```python
from build123d import *

# Parameters (mm, degrees)
SKETCH1_W           = 203.2
SKETCH1_H           = 247.65
BOSS_EXTRUDE1_DEPTH = 19.05
FILLET1_R           = 7.62
SHELL1_T            = -2.54
CUT_EXTRUDE1_REACH  = 163.301
SKETCH2_W           = 130.745
SKETCH2_H           = 180.34
FILLET2_R           = 2.54
CUT_EXTRUDE2_REACH  = 163.301
SKETCH3_R           = 2.54
SKETCH4_W           = 135.825
SKETCH4_H           = 185.42
CUT_EXTRUDE3_DEPTH  = 1.27


with BuildPart() as part:
    # Sketch1 → Boss-Extrude1 (new body)
    with BuildSketch(Plane(origin=(0, 0, 0), x_dir=(1, 0, 0), z_dir=(0, 1, 0))):
        Rectangle(SKETCH1_W, SKETCH1_H)
    extrude(amount=BOSS_EXTRUDE1_DEPTH)

    # Fillet1
    fillet1_edges = [part.edges().sort_by_distance(p)[0] for p in [
        (-101.6, 19.05, 0),
        (0, 19.05, 123.825),
        (101.6, 19.05, 0),
        (0, 19.05, -123.825),
    ]]
    fillet(fillet1_edges, radius=FILLET1_R)

    # Shell1
    shell1_openings = [part.faces().sort_by_distance(p)[0] for p in [
        (0, 0, 0),
    ]]
    offset(amount=SHELL1_T, openings=shell1_openings)

    # Sketch2 → Cut-Extrude1 (cut, up to next)
    with BuildSketch(Plane(origin=(0, 19.05, 0), x_dir=(1, 0, 0), z_dir=(0, 1, 0)), mode=Mode.PRIVATE) as cut_extrude1_sk1:
        with Locations((2.5725, 0)):
            Rectangle(SKETCH2_W, SKETCH2_H)
    cut_extrude1_tool1 = extrude(cut_extrude1_sk1.sketch, amount=-CUT_EXTRUDE1_REACH, mode=Mode.PRIVATE) & part.part
    add(cut_extrude1_tool1.solids().sort_by_distance((2.5725, 19.05, 0))[0], mode=Mode.SUBTRACT)

    # Fillet2
    fillet2_edges = [part.edges().sort_by_distance(p)[0] for p in [
        (-62.8, 19.05, 0),
        (2.5725, 19.05, 90.17),
        (67.945, 19.05, 0),
        (2.5725, 19.05, -90.17),
    ]]
    fillet(fillet2_edges, radius=FILLET2_R - 0.0001)  # a hair under: the kernel refuses the full size

    # Sketch3 → Cut-Extrude2 (cut, up to next)
    with BuildSketch(Plane(origin=(0, 19.05, 0), x_dir=(1, 0, 0), z_dir=(0, 1, 0)), mode=Mode.PRIVATE) as cut_extrude2_sk1:
        with Locations(Location((-85.725, 104.775, 0), (0, 0, 270))):
            Circle(SKETCH3_R)
    cut_extrude2_tool1 = extrude(cut_extrude2_sk1.sketch, amount=-CUT_EXTRUDE2_REACH, mode=Mode.PRIVATE) & part.part
    # Sketch3 → Cut-Extrude2 (cut, up to next)
    with BuildSketch(Plane(origin=(0, 19.05, 0), x_dir=(1, 0, 0), z_dir=(0, 1, 0)), mode=Mode.PRIVATE) as cut_extrude2_sk2:
        with Locations(Location((-85.725, -104.775, 0), (0, 0, 270))):
            Circle(SKETCH3_R)
    cut_extrude2_tool2 = extrude(cut_extrude2_sk2.sketch, amount=-CUT_EXTRUDE2_REACH, mode=Mode.PRIVATE) & part.part
    add(cut_extrude2_tool1.solids().sort_by_distance((-85.725, 19.05, -104.775))[0], mode=Mode.SUBTRACT)
    add(cut_extrude2_tool2.solids().sort_by_distance((-85.725, 19.05, 104.775))[0], mode=Mode.SUBTRACT)

    # Sketch4 → Cut-Extrude3 (cut)
    with BuildSketch(Plane.XZ.offset(-16.51)):
        with Locations((2.5725, 0)):
            Rectangle(SKETCH4_W, SKETCH4_H)
    extrude(amount=-CUT_EXTRUDE3_DEPTH, mode=Mode.SUBTRACT)


solid = part.part
```
Input: part model. Units: mm. Frame: model coordinates. A direction names the side the tool comes from. Coordinates: 2 decimals unless noted, no trailing zeros. Write each loop counter-clockwise with the first axis right and the second up, starting at its lowest first coordinate (ties: lowest second). Pieces come first, ordered by that corner, then holes. Notation, with made-up numbers: (27.5, -22) -> (47.5, -22) arc R27 cw to (47.5, 11) -> close; hole circle Ø5 at (47, -18). An arc over 180 degrees is marked (long way). Write each question's results on one line, items separated by ' | '.
Item 1: Section query B-B on y = 3. Return loops of the section in (x, z) (3 decimals).
Conclusion:
outline: (-101.6, -123.825) -> (101.6, -123.825) -> (101.6, 123.825) -> (-101.6, 123.825) -> close; hole (-99.06, -121.285) -> (99.06, -121.285) -> (99.06, 121.285) -> (-99.06, 121.285) -> close
Item 2: Section query C-C on x = -5. Return loops of the section in (y, z) (3 decimals), plus the area to 3 significant figures.
Conclusion:
outline: (0, -123.825) -> (11.43, -123.825) arc R7.62 ccw to (19.05, -116.205) -> (19.05, -92.71) arc R2.54 ccw to (17.78, -90.51) -> (17.78, -92.71) -> (16.51, -92.71) -> (16.51, -116.205) arc R5.08 cw to (11.43, -121.285) -> (0, -121.285) -> close; (0, 121.285) -> (11.43, 121.285) arc R5.08 cw to (16.51, 116.205) -> (16.51, 92.71) -> (17.78, 92.71) -> (17.78, 90.51) arc R2.54 ccw to (19.05, 92.71) -> (19.05, 116.205) arc R7.62 ccw to (11.43, 123.825) -> (0, 123.825) -> close | area: 232 mm^2
Item 3: Material intervals for probe 1 along X at (y, z) = (6, 113); probe 2 along Z at (x, y) = (86, 11) (3 decimals); probe 3 along Y at (x, z) = (27.5, 98), sorted ascending.
Conclusion:
probe 1: x = -101.6 to -99.06, 99.06 to 101.6 | probe 2: z = -123.825 to -121.285, 121.285 to 123.825 | probe 3: y = 16.51 to 19.05
Item 4: Mould query, pull axis X, two halves, no side actions, for faces 1 (the flat face through (-99.06, 6, 2)), 2 (the flat face through (-1, 6, -121.285)), 3 (the flat face through (-101.6, 6, 2)), 4 (the cylindrical face through (1.42, 16.76, -121.65)). Classes: +X half, -X half, draft (parallel to the pull), parting line (faces both ways), or undercut.
Conclusion:
face 1: undercut | face 2: undercut | face 3: -X half | face 4: draft
Item 5: Pin query (flat end, axial travel): pin 1 Ø3 at (x, z) = (-85.725, -104.775) entering from +Y; pin 2 Ø0.6 at (x, y) = (-2, 17) entering from +Z; pin 3 Ø1.4 at (y, z) = (17.5, -3) entering from -X; pin 4 Ø3 at (x, y) = (4.5, 14) entering from +Z. Return the tip coordinate at first contact, or that it passes through.
Conclusion:
pin 1: passes through | pin 2: stops at z = 121.71 | pin 3: stops at x = -99.39 | pin 4: stops at z = 123.75
Item 6: Section query A-A on z = -15.5. Return loops of the section in (x, y) (3 decimals).
Conclusion:
outline: (-101.6, 0) -> (-99.06, 0) -> (-99.06, 11.43) arc R5.08 cw to (-93.98, 16.51) -> (-65.34, 16.51) -> (-65.34, 17.78) -> (-63.14, 17.78) arc R2.54 ccw to (-65.34, 19.05) -> (-93.98, 19.05) arc R7.62 ccw to (-101.6, 11.43) -> close; (68.285, 17.78) -> (70.485, 17.78) -> (70.485, 16.51) -> (93.98, 16.51) arc R5.08 cw to (99.06, 11.43) -> (99.06, 0) -> (101.6, 0) -> (101.6, 11.43) arc R7.62 ccw to (93.98, 19.05) -> (70.485, 19.05) arc R2.54 ccw to start
Item 7: Set-up query: faces 5 (the flat face through (99.06, 6, 2)), 6 (the cylindrical face through (-99.427, 16.759, -1.734)). Return all of +Z, -Z, +X, -X, +Y, -Y with unobstructed straight access to the full face (end or side cutting, diameter ignored); none if empty.
Conclusion:
face 5: -Y | face 6: +Z, -Z, -X, +Y
Item 8: Section query D-D on x = 77. Return loops of the section in (y, z) (3 decimals).
Conclusion:
outline: (0, -123.825) -> (11.43, -123.825) arc R7.62 ccw to (19.05, -116.205) -> (19.05, 116.205) arc R7.62 ccw to (11.43, 123.825) -> (0, 123.825) -> (0, 121.285) -> (11.43, 121.285) arc R5.08 cw to (16.51, 116.205) -> (16.51, -116.205) arc R5.08 cw to (11.43, -121.285) -> (0, -121.285) -> close
